from build123d import *

# Parameters (mm, degrees)
F0_R     = 12.5
F1_DEPTH = 10
F2_R     = 9.05
F2_R_2   = 3.75
F3_DEPTH = 1
F4_DEPTH = 7.5


with BuildPart() as f1:
    # F0 (on Top) → F1 (new body)
    with BuildSketch(Plane.XY):
        with BuildLine():
            ThreePointArc((0, 17.5), (5.125631, 5.125631), (17.5, 0))
            Line((17.5, 0), (53, 0))
            ThreePointArc((53, 0), (56.535534, 1.464466), (58, 5))
            Line((58, 5), (58, 30))
            ThreePointArc((58, 30), (56.535534, 33.535534), (53, 35))
            Line((53, 35), (17.5, 35))
            ThreePointArc((17.5, 35), (5.125631, 29.874369), (0, 17.5))
        make_face()
        with Locations((17.5, 17.5)):
            Circle(F0_R, mode=Mode.SUBTRACT)
    extrude(amount=F1_DEPTH)

    # F2 (on face) → F3 (join)
    with BuildSketch(Plane.XY.offset(10)):
        with Locations((44, 17.5)):
            Circle(F2_R)
        with Locations((44, 17.5)):
            Circle(F2_R_2, mode=Mode.SUBTRACT)
    extrude(amount=F3_DEPTH)

    # F2 (on face) → F4 (cut)
    with BuildSketch(Plane.XY.offset(10)):
        with Locations((44, 17.5)):
            Circle(F2_R_2)
    extrude(amount=-F4_DEPTH, mode=Mode.SUBTRACT)


solid = f1.part
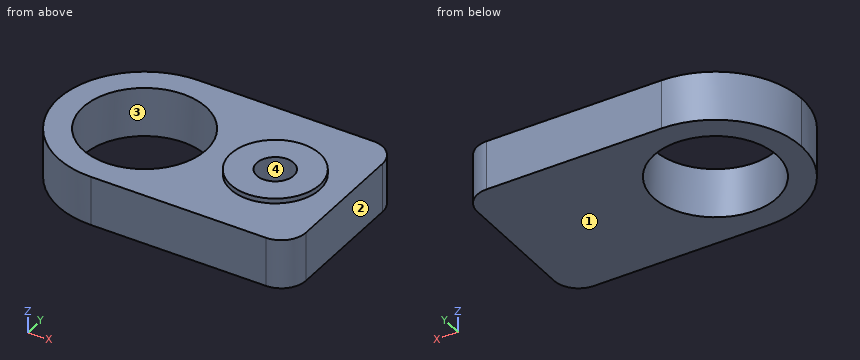
Model file for the job. Use its own axes, mm. Face numbers are marked on the shaded views. Coordinates: 2 decimals unless noted, no trailing zeros. Order: outer loops, then holes, each group sorted by start corner. A loop starts at its lowest first (then second) coordinate and runs counter-clockwise, first axis right, second up. Notation, with made-up numbers: (-23, 54) -> (5, 54) arc R19 cw to (5, 90) -> close; hole circle Ø9 at (-31.75, 22.25). An arc over 180 degrees is marked (long way). Return JSON: item names as keys, results as strings. Group by question number.
Item 1: Pull direction X, two halves, no side cores. Call the marked faces 1, 2, 3 and 4: pulls with the +X half, pulls with the -X half, needs draft (parallel to the pull), parting line crosses it, or undercut.
Item 2: Wall check: line 1 along Y through (x, z) = (17.5, 4.75); line 2 along Y through (x, z) = (44, 6); line 3 along Z through (x, y) = (34, 28). Give the ranges that are in metal, low to high. Write a range as [from, to].
Item 3: Saw through at D-D on x = 44. Write the cut outline in (y, z).
Item 4: Saw through at B-B on z = 6.75. Write the cut outline in (x, y).
Item 5: Saw through at A-A on y = 10.5. Write the cut outline in (x, z), then the cut area to 3 significant figures.
Item 6: Saw through at C-C on x = 24. Write the cut outline in (y, z).
Item 7: Flat gauge pins, fed straight in: P1, Ø7, axis at x = 44, y = 17.5, coming from the -Z side; P2, Ø17.5, axis at x = 23, y = 12.5, coming from the +Z side; P3, Ø3, axis at y = 15.5, z = 9.5, coming from the -X side; P4, Ø15, axis at x = 17.5, y = 17.5, coming from the +Z side. Where does each tip first touch, or does it go through?
Values found:
{
 "1": {"face 1": "needs draft", "face 2": "pulls with the +X half", "face 3": "undercut", "face 4": "undercut"},
 "2": {"line 1": "y = [0, 5], [30, 35]", "line 2": "y = [0, 13.75], [21.25, 35]", "line 3": "z = [0, 10]"},
 "3": {"outline": "(0, 0) -> (35, 0) -> (35, 10) -> (26.55, 10) -> (26.55, 11) -> (21.25, 11) -> (21.25, 2.5) -> (13.75, 2.5) -> (13.75, 11) -> (8.45, 11) -> (8.45, 10) -> (0, 10) -> close"},
 "4": {"outline": "(0, 17.5) arc R17.5 ccw to (17.5, 0) -> (53, 0) arc R5 ccw to (58, 5) -> (58, 30) arc R5 ccw to (53, 35) -> (17.5, 35) arc R17.5 ccw to start; hole circle Ø25 at (17.5, 17.5); hole circle Ø7.5 at (44, 17.5)"},
 "5": {"outline": "(1.46, 0) -> (7.14, 0) -> (7.14, 10) -> (1.46, 10) -> close; (27.86, 0) -> (58, 0) -> (58, 10) -> (49.74, 10) -> (49.74, 11) -> (38.26, 11) -> (38.26, 10) -> (27.86, 10) -> close", "area": "370 mm2"},
 "6": {"outline": "(0, 0) -> (6.82, 0) -> (6.82, 10) -> (0, 10) -> close; (28.18, 0) -> (35, 0) -> (35, 10) -> (28.18, 10) -> close"},
 "7": {"P1": "stops at z = 0", "P2": "stops at z = 10", "P3": "stops at x = 0.01", "P4": "passes through"}
}
